Part print with two shaded views. Sizes in mm from the minimum x, y, z corner. Coordinates: 2 decimals unless noted, no trailing zeros.
Q1. Pin check, flat tip, straight feed: P1, Ø2, axis at x = 8, y = 7, coming from the +Z side. Stop position of the tip, or through.
Q2. Pull direction Y, two halves, no side cores. Call the marked faces 1, 2 and 3: released by +Y, released by -Y, zero draft, split by the parting line, or undercut.
Q3. Drill centre lines: probe 1 along Z at (x, y) = (54, 10); probe 2 along X at (y, z) = (11, 51.5); probe 3 along Z at (x, y) = (5.5, 16.25). Where is each one in solid material? Low to high.
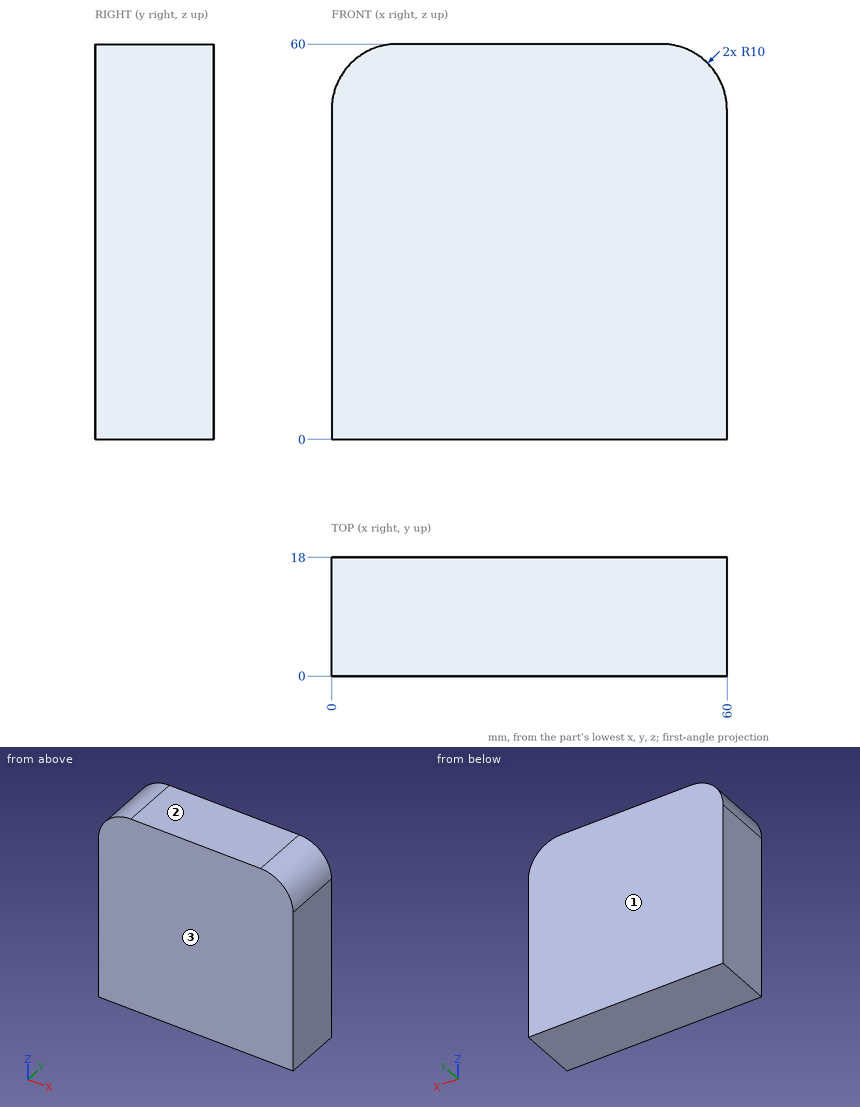
Answer sheet:
1. P1: stops at z = 59.95
2. face 1: released by +Y
2. face 2: zero draft
2. face 3: released by -Y
3. probe 1: z = 0 to 59.17
3. probe 2: x = 0.11 to 59.89
3. probe 3: z = 0 to 58.93
